Source: three-view drawing plus pictorial views. Frame: mm from the lowest corner of the part. Give positions to 0.01 mm unless a question says otherwise; leave off trailing zeros. Write each loop counter-clockwise with the first axis right and the second up, starting at its lowest first coordinate (ties: lowest second). Pieces come first, ordered by that corner, then holes. Notation, with made-up numbers: (16.25, 44.25) -> (59.25, 44.25) arc R10 ccw to (59.25, 61.25) -> close; hole circle Ø6 at (31.25, 77.25). An arc over 180 degrees is marked (long way). Answer in a Markdown table with one row per item. Add a question column.
Item 1: Section query B-B on y = 26. Output: boundary loops of the cut face in (x, z), plus the area to 3 significant figures.
Item 2: Section query C-C on x = 18.5. Output: boundary loops of the cut face in (y, z), plus the area to 3 significant figures.
Item 3: Section query A-A on z = 1.65. State how many separate pieces and enclosed holes the cut face has, plus the area to 3 significant figures.
Item 4: First-contact query: P1, Ø1, axis at x = 136, z = 4, coming from the +Y side; P2, Ø2.5, axis at x = 58.5, z = 2.5, coming from the -Y side; P3, Ø2, axis at y = 41.5, z = 3, coming from the +X side; P4, Ø2, axis at y = 130.5, z = 2, coming from the -X side. Flat tips, straight axial feed; report the tip coordinate or a pass-through.
Item 5: Material intervals for probe 1 along X at (y, z) = (86.3, 3.2); probe 2 along X at (y, z) = (91, 1); probe 3 along X at (y, z) = (169.1, 1.6), sorted ascending. Write a range as from..to.
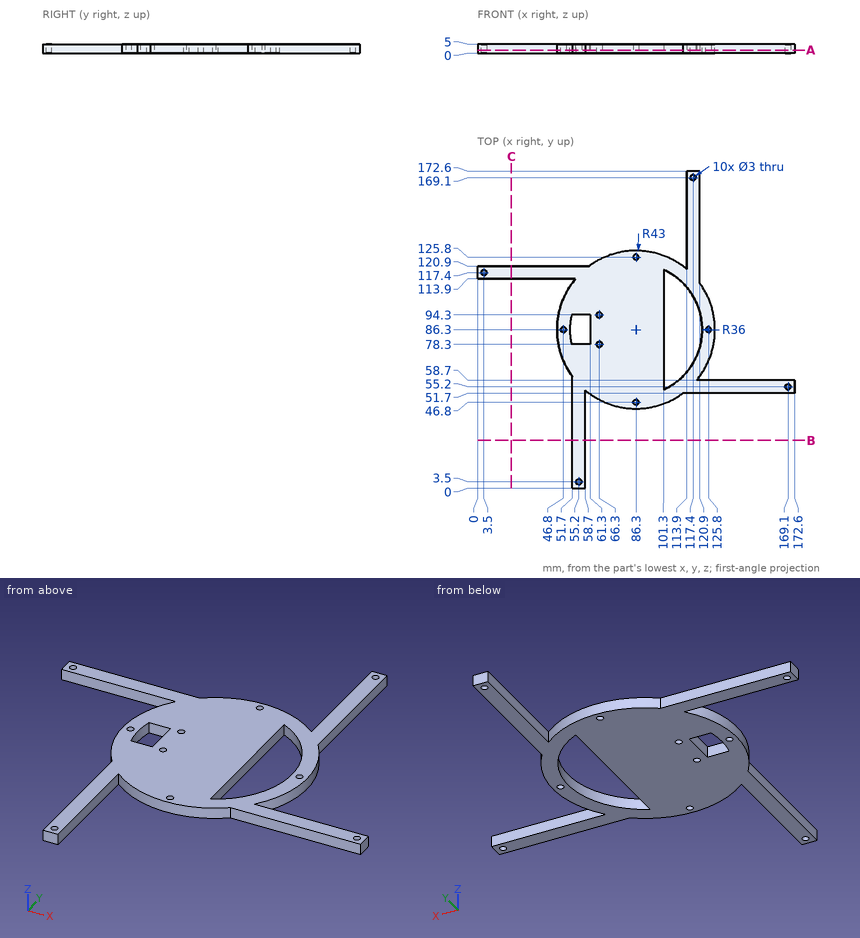
Findings below:
| question | item | result |
|---|---|---|
| 1 | outline | (51.7, 0) -> (58.7, 0) -> (58.7, 5) -> (51.7, 5) -> close |
| 1 | area | 35.0 mm^2 |
| 2 | outline | (113.9, 0) -> (120.9, 0) -> (120.9, 5) -> (113.9, 5) -> close |
| 2 | area | 35.0 mm^2 |
| 3 | separate pieces | 1 |
| 3 | enclosed holes | 12 |
| 3 | area | 6,170 mm^2 |
| 4 | P1 | stops at y = 58.7 |
| 4 | P2 | stops at y = 0 |
| 4 | P3 | stops at x = 58.7 |
| 4 | P4 | stops at x = 113.9 |
| 5 | probe 1 | x = 43.3..45.3, 48.3..50.3, 61.3..101.3, 122.3..124.3, 127.3..129.3 |
| 5 | probe 2 | x = 43.56..50.61, 61.3..101.3, 121.99..129.04 |
| 5 | probe 3 | x = 113.9..115.9, 118.9..120.9 |
